Source: CAD feature listing. Evaluate the final solid. Frame: model axes, mm. Face numbers are marked on the shaded views. A direction names the side the tool comes from. Coordinates: 2 decimals unless noted, no trailing zeros. Order: outer loops, then holes, each group sorted by start corner. A loop starts at its lowest first (then second) coordinate and runs counter-clockwise, first axis right, second up. Notation, with made-up numbers: (33, 24.25) -> (73, 24.25) arc R25 cw to (73, 58.25) -> close; hole circle Ø4 at (58, 69). An arc over 180 degrees is marked (long way). Put each result on its own line as item: value.
Autodesk Inventor part; units mm, degrees
ref_plane "YZ Plane" through (0, 0, 0) normal (1, 0, 0) x (0, 1, 0)
ref_plane "XZ Plane" through (0, 0, 0) normal (0, 1, 0) x (-1, 0, 0)
ref_plane "XY Plane" through (0, 0, 0) normal (0, 0, 1) x (1, 0, 0)
sketch "Sketch1" plane through (0, 0, 0) normal (0, 1, 0) x (-1, 0, 0)
  line L0 (12.65, 7.65) -> (-12.65, 7.65)
  line L1 (-12.65, 7.65) -> (-12.65, -7.65)
  line L2 (-12.65, -7.65) -> (12.65, -7.65)
  line L3 (12.65, -7.65) -> (12.65, 7.65)
  point P0 (0, 0)
  point P1 (0, 7.65)
  point P2 (12.65, 0)
  dimension "d0" = 15.3
  dimension "d1" = 25.3
extrude "Extrusion1" add sketch "Sketch1" along normal blind 10
sketch "Sketch2" plane through (0, 10, 0) normal (0, 1, 0) x (1, 0, 0)
  line L0 (-12.65, -7.65) -> (12.65, -7.65)
  line L1 (12.65, -7.65) -> (12.65, 7.65)
  line L2 (12.65, 7.65) -> (-12.65, 7.65)
  line L3 (-12.65, 7.65) -> (-12.65, -7.65)
  line L4 (19, 15) -> (-19, 15)
  line L5 (-19, 15) -> (-19, -15)
  line L6 (-19, -15) -> (19, -15)
  line L7 (19, -15) -> (19, 15)
  point P0 (0, 0)
  point P1 (19, 0)
  point P2 (0, 15)
  dimension "d4" = 30
  dimension "d5" = 38
extrude "Extrusion2" add sketch "Sketch2" along normal blind 8 contours L3 L2 L1 L0 | L7 L6 L5 L4
sketch "Sketch3" plane through (0, 18, 0) normal (0, 1, 0) x (1, 0, 0)
  line L0 (19, 15) -> (-19, 15)
  line L1 (-19, 15) -> (-19, -15)
  line L2 (-19, -15) -> (19, -15)
  line L3 (19, -15) -> (19, 15)
  line L4 (-19, -14) -> (9, -14)
  line L5 (9, -14) -> (9, 14)
  line L6 (9, 14) -> (-19, 14)
  line L7 (-19, 14) -> (-19, -14)
  line L8 (-19, -14) -> (-19, 0) construction
  line L9 (-19, 0) -> (9, 0) construction
  point P0 (0, 0)
  point P1 (-19, 0)
  point P2 (-5, 0)
  dimension "d8" = 28
  dimension "d9" = 28
  dimension "d10" = 14
extrude "Extrusion3" add sketch "Sketch3" along normal blind 9 contours L6 L5 L4 L1
properties part number "Modulo"
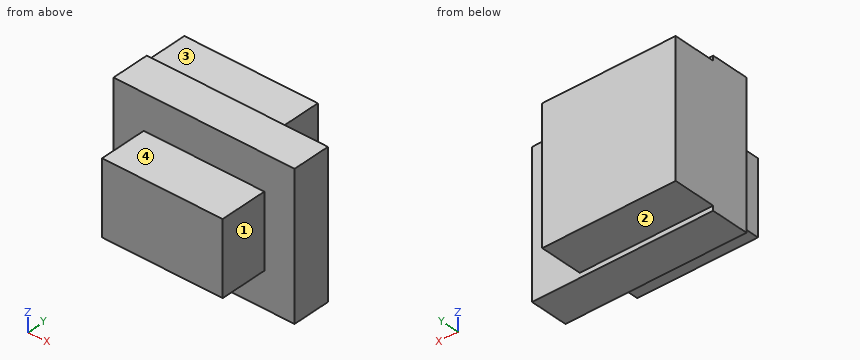
1. Set-up query: the marked faces 1, 2, 3 and 4. Return all of +Z, -Z, +X, -X, +Y, -Y with unobstructed straight access to the full face (end or side cutting, diameter ignored); none if empty.
Numbers:
face 1: +Z, -Z, +X, -Y
face 2: -Z, +X, -X, +Y
face 3: +Z, +X, -X, +Y
face 4: +Z, +X, -X, -Y
2. First-contact query: pin 1 (7 mm diameter, centred on y = 22.5, z = -3, fed in from +X); pin 2 (3 mm diameter, centred on y = 5, z = 3, fed in from +X); pin 3 (11 mm diameter, centred on y = 2.5, z = 1, fed in from -X). Flat tips, straight axial feed; report the tip coordinate or a pass-through.
Numbers:
pin 1: stops at x = 9
pin 2: stops at x = 12.65
pin 3: stops at x = -12.65
3. Cut plane C-C on y = 19.75. Output: boundary loops of the cut face in (x, z).
Numbers:
outline: (-19, -14) -> (9, -14) -> (9, 14) -> (-19, 14) -> close
4. Cut plane B-B on z = 1.25. Output: boundary loops of the cut face in (x, y), plus the area to 3 significant figures.
Numbers:
outline: (-19, 10) -> (-12.65, 10) -> (-12.65, 0) -> (12.65, 0) -> (12.65, 10) -> (19, 10) -> (19, 18) -> (9, 18) -> (9, 27) -> (-19, 27) -> close
area: 809 mm2
5. Ray query, line 1 along X through (y, z) = (21.25, 4.75); line 2 along Y through (x, z) = (15, -1.5); line 3 along Y through (x, z) = (-2, 10.5). Return the intervals inside material, ascending.
Numbers:
line 1: x = -19 to 9
line 2: y = 10 to 18
line 3: y = 10 to 27
6. Cut plane D-D on z = 8.5. Output: boundary loops of the cut face in (x, y), plus the area to 3 significant figures.
Numbers:
outline: (-19, 10) -> (19, 10) -> (19, 18) -> (9, 18) -> (9, 27) -> (-19, 27) -> close
area: 556 mm2
7. Cut plane A-A on x = -14.5. Output: boundary loops of the cut face in (y, z), plus the area to 3 significant figures.
Numbers:
outline: (10, -15) -> (18, -15) -> (18, -14) -> (27, -14) -> (27, 14) -> (18, 14) -> (18, 15) -> (10, 15) -> close
area: 492 mm2
